For this review, use the dimensioned drawing (mm, ordinates from the lowest corner) and the shaded views. A direction names the side the tool comes from. Give positions to 0.01 mm unless a question says otherwise; leave off trailing zeros. Order: outer loops, then holes, each group sorted by start corner. A loop starts at its lowest first (then second) coordinate and runs counter-clockwise, first axis right, second up.
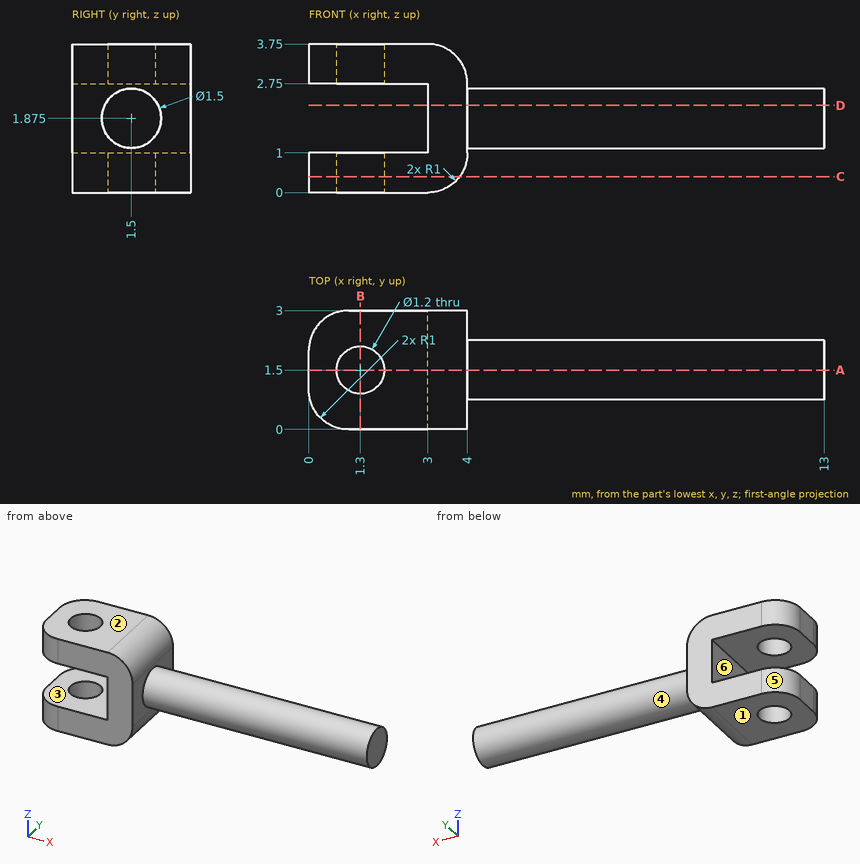
1. Machinability: for the marked faces 4, 5 and 6, which of the approach directions +Z, -Z, +X, -X, +Y, -Y give a long, thin tool a straight path to every point of the face, cutting with its end or side? Answer none if there is none.
Recorded:
face 4: +X
face 5: +Z, -Z, -X, +Y
face 6: -X, +Y, -Y
2. For line 1 along Z through (x, y) = (1.5, 2.55); line 2 along Y through (x, z) = (1.3, 3.4); line 3 along X through (y, z) = (2.3, 2.05), list the stretches that pass through material, from the lowest coordinate up.
Recorded:
line 1: z = 0 to 1, 2.75 to 3.75
line 2: y = 0 to 0.9, 2.1 to 3
line 3: x = 3 to 4
3. Draft analysis for pull direction Z (two halves, no side actions). For the marked faces 1, 2 and 3, state which applies: pulls with the +Z half, pulls with the -Z half, needs draft (parallel to the pull), parting line crosses it, or undercut.
Recorded:
face 1: pulls with the -Z half
face 2: pulls with the +Z half
face 3: undercut
4. Take a section at C-C (z = 0.4). State the section outline as (x, y) points.
Recorded:
outline: (0, 1) arc R1 ccw to (1, 0) - (3.8, 0) - (3.8, 3) - (1, 3) arc R1 ccw to (0, 2) - close; hole circle Ø1.2 at (1.3, 1.5)
5. Take a section at A-A (y = 1.5). State the section outline as (x, z) points (3 decimals), then the cut area to 3 significant figures.
Recorded:
outline: (0, 0) - (0.7, 0) - (0.7, 1) - (0, 1) - close; (0, 2.75) - (0.7, 2.75) - (0.7, 3.75) - (0, 3.75) - close; (1.9, 0) - (3, 0) arc R1 ccw to (4, 1) - (4, 1.125) - (13, 1.125) - (13, 2.625) - (4, 2.625) - (4, 2.75) arc R1 ccw to (3, 3.75) - (1.9, 3.75) - (1.9, 2.75) - (3, 2.75) - (3, 1) - (1.9, 1) - close
area: 20.4 mm2
6. Take a section at B-B (x = 1.3). State the section outline as (y, z) points, then the cut area to 3 significant figures.
Recorded:
outline: (0, 0) - (0.9, 0) - (0.9, 1) - (0, 1) - close; (0, 2.75) - (0.9, 2.75) - (0.9, 3.75) - (0, 3.75) - close; (2.1, 0) - (3, 0) - (3, 1) - (2.1, 1) - close; (2.1, 2.75) - (3, 2.75) - (3, 3.75) - (2.1, 3.75) - close
area: 3.60 mm2
7. For pin 1 (1.5 mm diameter, centred on x = 10, y = 2.5, fed in from +Z); pin 2 (2 mm diameter, centred on x = 8.5, z = 0.5, fed in from -Y), all flat-tipped, find the tip position at first contact; note any pin that passes through.
Recorded:
pin 1: stops at z = 2.58
pin 2: stops at y = 0.85
8. Take a section at D-D (z = 2.2). State the section outline as (x, y) points, then the cut area to 3 significant figures.
Recorded:
outline: (3, 0) - (4, 0) - (4, 0.82) - (13, 0.82) - (13, 2.18) - (4, 2.18) - (4, 3) - (3, 3) - close
area: 15.2 mm2
